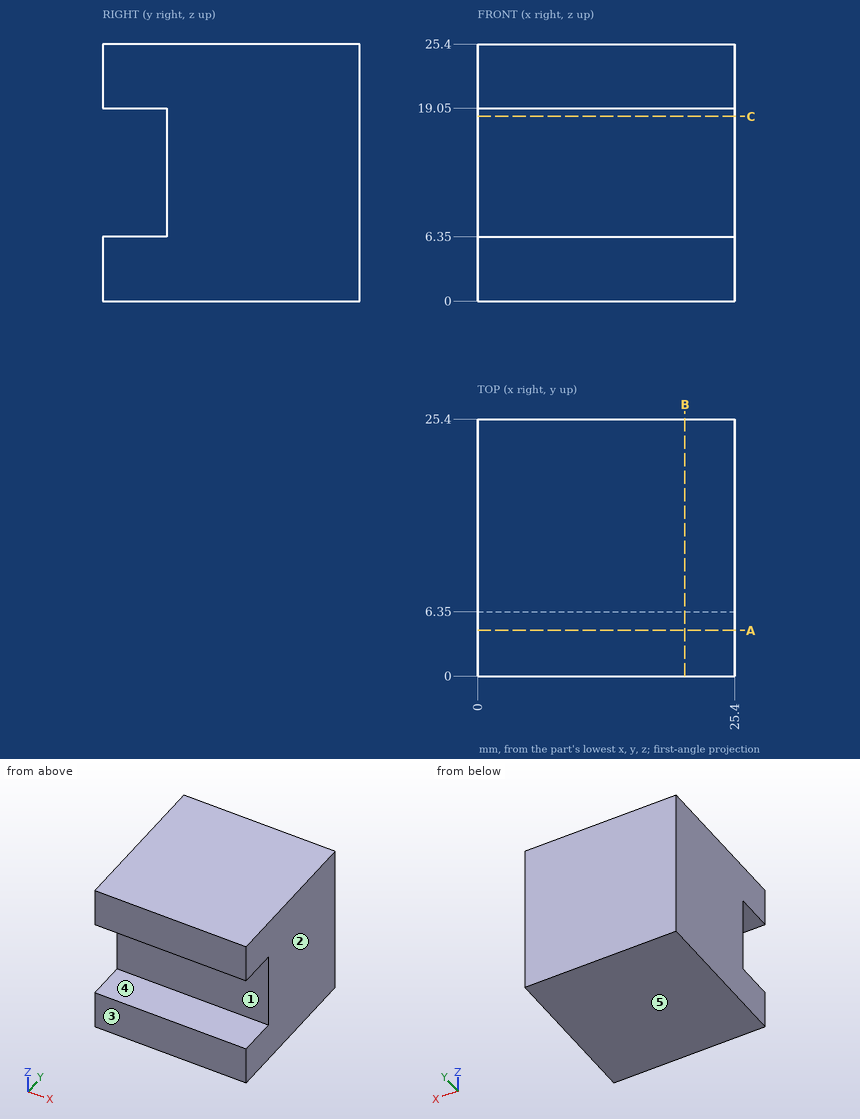
Verification items for this drawing (mm, ordinates from the low corner). A direction names the side the tool comes from. Coordinates: 2 decimals unless noted, no trailing zeros. Loops run counter-clockwise (first coordinate to the right, second up) from the corner with the lowest first, then second, coordinate; pieces in that order, holes last.
Item 1: Sectioned sample at A-A, the plane y = 4.5. Record the boundary of the cut face in (x, z).
Item 2: Sectioned sample at C-C, the plane z = 18.25. Record the boundary of the cut face in (x, y), then the cut area to 3 significant figures.
Item 3: Sectioned sample at B-B, the plane x = 20.5. Record the boundary of the cut face in (y, z).
Item 4: Access from +Z, -Z, +X, -X, +Y, -Y to the whole of each face (thin tool, end or side, straight path). Record for the marked faces 1 and 2.
Item 5: Go/stop test with a flat-tipped pin: pin 1 Ø6.5 at (x, z) = (7, 12) entering from -Y. Record where the tip stops, or that it passes through.
Item 6: Release check for a two-part mould opening along Z. For the marked faces 3, 4 and 5 record: released by +Z, released by -Z, zero draft, split by the parting line, or undercut.
Item 7: Thickness scan on line 1 (Y direction, x = 22.75, z = 14.25); line 2 (Z direction, x = 3.5, y = 1). Record the ranges inside material, lowest first.
Check result:
1. outline: (0, 0) - (25.4, 0) - (25.4, 6.35) - (0, 6.35) - close; (0, 19.05) - (25.4, 19.05) - (25.4, 25.4) - (0, 25.4) - close
2. outline: (0, 6.35) - (25.4, 6.35) - (25.4, 25.4) - (0, 25.4) - close
2. area: 484 mm2
3. outline: (0, 0) - (25.4, 0) - (25.4, 25.4) - (0, 25.4) - (0, 19.05) - (6.35, 19.05) - (6.35, 6.35) - (0, 6.35) - close
4. face 1: +X, -X, -Y
4. face 2: +Z, -Z, +X, +Y, -Y
5. pin 1: stops at y = 6.35
6. face 3: zero draft
6. face 4: undercut
6. face 5: released by -Z
7. line 1: y = 6.35 to 25.4
7. line 2: z = 0 to 6.35, 19.05 to 25.4
